from build123d import *

# Parameters (mm, degrees)
SKETCH1_R           = 5.5
SKETCH1_R_2         = 4.5
SKETCH1_R_3         = 4
BOSS_EXTRUDE1_DEPTH = 1
SKETCH1_3_R         = 4
BOSS_EXTRUDE2_DEPTH = 16
SKETCH2_R           = 1.5
CUT_EXTRUDE1_DEPTH  = 13
SKETCH1_4_R         = 4.5
SKETCH1_4_R_2       = 4
BOSS_EXTRUDE3_DEPTH = 25
BOSS_EXTRUDE4_START = 24
SKETCH1_5_R         = 5.5
SKETCH1_5_R_2       = 4.5
BOSS_EXTRUDE4_DEPTH = 1
SKETCH5_R           = 1.5
CUT_EXTRUDE2_DEPTH  = 11.5


with BuildPart() as part:
    # Sketch1 → Boss-Extrude1 (new body)
    with BuildSketch(Plane(origin=(0, 0, 0), x_dir=(1, 0, 0), z_dir=(0, 1, 0))):
        Circle(SKETCH1_R)
        Circle(SKETCH1_R_2, mode=Mode.SUBTRACT)
        Circle(SKETCH1_R_2)
        Circle(SKETCH1_R_3, mode=Mode.SUBTRACT)
        Circle(SKETCH1_R_3)
    extrude(amount=BOSS_EXTRUDE1_DEPTH)

    # Sketch1_3 → Boss-Extrude2 (add)
    with BuildSketch(Plane(origin=(0, 0, 0), x_dir=(1, 0, 0), z_dir=(0, 1, 0))):
        Circle(SKETCH1_3_R)
    extrude(amount=-BOSS_EXTRUDE2_DEPTH)

    # Sketch2 → Cut-Extrude1 (cut)
    with BuildSketch(Plane(origin=(4, 0, 0), x_dir=(0, 0, -1), z_dir=(1, 0, 0))):
        with Locations((0, -13)):
            Circle(SKETCH2_R)
    extrude(amount=-CUT_EXTRUDE1_DEPTH, mode=Mode.SUBTRACT)

    # Sketch1_4 → Boss-Extrude3 (add)
    with BuildSketch(Plane(origin=(0, 0, 0), x_dir=(1, 0, 0), z_dir=(0, 1, 0))):
        Circle(SKETCH1_4_R)
        Circle(SKETCH1_4_R_2, mode=Mode.SUBTRACT)
    extrude(amount=BOSS_EXTRUDE3_DEPTH)

    # Sketch1_5 → Boss-Extrude4 (add)
    with BuildSketch(Plane(origin=(0, 0, 0), x_dir=(1, 0, 0), z_dir=(0, 1, 0)).offset(BOSS_EXTRUDE4_START)):
        Circle(SKETCH1_5_R)
        Circle(SKETCH1_5_R_2, mode=Mode.SUBTRACT)
    extrude(amount=BOSS_EXTRUDE4_DEPTH)

    # Sketch5 → Cut-Extrude2 (cut, symmetric)
    with BuildSketch(Plane(origin=(4, 0, 0), x_dir=(0, 0, -1), z_dir=(1, 0, 0))):
        with Locations((0, 15)):
            Circle(SKETCH5_R)
    extrude(amount=CUT_EXTRUDE2_DEPTH, both=True, mode=Mode.SUBTRACT)


solid = part.part
Read the model definition and answer for the solid it produces. Units are mm, in the model's axes. A direction names the side the tool comes from. Give positions to 0.01 mm unless a question says otherwise; leave off trailing zeros. Loops run counter-clockwise (first coordinate to the right, second up) from the corner with the lowest first, then second, coordinate; pieces in that order, holes last. Notation, with made-up numbers: M 49.25,9 L 55.25,9 A21 ccw 55.25,14 Z; hole C -26,37.25 d8. An arc over 180 degrees is marked long. Write each question's results on one line, items separated by ' | '.
1. Straight lines are drawn through the part: line 1 (Y direction, x = -0.5, z = 0); line 2 (Z direction, x = 0, y = 7); line 3 (Y direction, x = 3.5, z = 4). For each, find the intervals that lie inside material, in ascending order. Write a range as [from, to].
Values:
line 1: y = [-16, -14.5], [-11.5, 1] | line 2: z = [-4.5, -4], [4, 4.5] | line 3: y = [0, 1], [24, 25]
2. Section B-B on x = 0 is taken. Give the vertices of the cut face in (y, z).
Values:
outline: M -16,-4 L 0,-4 L 0,-5.5 L 1,-5.5 L 1,-4.5 L 24,-4.5 L 24,-5.5 L 25,-5.5 L 25,-4 L 1,-4 L 1,4 L 25,4 L 25,5.5 L 24,5.5 L 24,4.5 L 1,4.5 L 1,5.5 L 0,5.5 L 0,4 L -16,4 Z; hole C -13,0 d3
3. The mould has two halves that part along Z. Classify faces 4 (the face through (-4.1, 15.45, -1.43)), 5 (the face through (-4, 0, 2)), 6 (the face through (4.11, 16.01, 1.11)), 7 (the face through (-1.19, 24.49, 5.37)): pulls with the +Z half, pulls with the -Z half, needs draft (parallel to the pull), parting line crosses it, or undercut.
Values:
face 4: undercut | face 5: needs draft | face 6: undercut | face 7: parting line crosses it
4. Section D-D on y = 23.5 is taken. Give the vertices of the cut face in (x, z).
Values:
outline: C 0,0 d9; hole C 0,0 d8
5. Given pin 1 (3 mm diameter, centred on y = 9, z = -2.5, fed in from -X); pin 2 (4 mm diameter, centred on y = -5.5, z = -1.5, fed in from +X); pin 3 (4 mm diameter, centred on y = 15, z = 0, fed in from -X); pin 4 (5.5 mm diameter, centred on x = -2.5, z = 1, fed in from +Y), each flat-ended and moving along its own axis, determine where each tip first touches the part or whether it passes through.
Values:
pin 1: stops at x = -4.39 | pin 2: stops at x = 4 | pin 3: stops at x = -4.5 | pin 4: stops at y = 25
6. Section A-A on z = 0 is taken. State how many separate pieces and enclosed holes the cut face has, plus the area to 3 significant figures.
Values:
separate pieces: 4 | enclosed holes: 0 | area: 138 mm^2
7. Section C-C on y = -13 is taken. Give the vertices of the cut face in (x, z), plus the area to 3 significant figures.
Values:
outline: M -3.71,-1.5 A4 ccw 3.71,-1.5 Z; M -3.71,1.5 L 3.71,1.5 A4 ccw Z | area: 26.8 mm^2
8. A tool of negligible diameter and unlimited length cuts with its end or side. For faces 1 (the face through (1.846, -7.888, 3.549)), 2 (the face through (-0.867, 12.832, 3.905)), 3 (the face through (-5, 1, 0)), from which of +Z, -Z, +X, -X, +Y, -Y can it reach the whole face along a straight path? Write none if from no direction.
Values:
face 1: -Y | face 2: +Y | face 3: none
